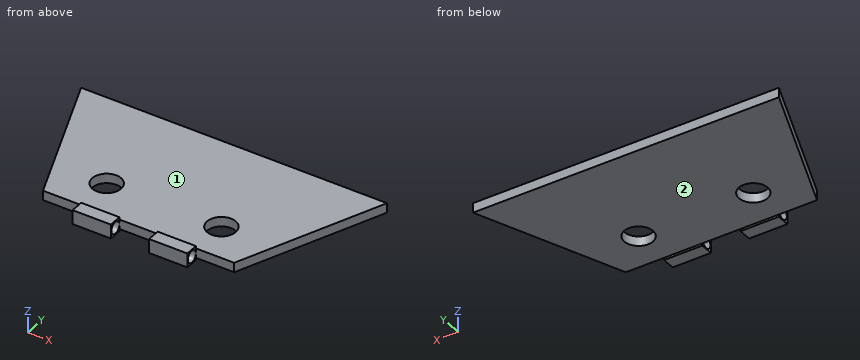
```python
from build123d import *

# Parameters (mm, degrees)
F1_DEPTH = 6.35
F2_W     = 8.614382
F2_H     = 9.368035
F2_R     = 3.988724
F3_DEPTH = 76.2
F4_W     = 25.4
F4_H     = 8.614382
F5_DEPTH = 25.4
F8_D     = 19.05


with BuildPart() as f1:
    # F0 (on Top) → F1 (new body)
    with BuildSketch(Plane.XY):
        Polygon((139.7, 95.249673), (-63.5, 95.249673), (-25.4, 0), (101.6, 0), align=None)
    extrude(amount=F1_DEPTH)

    # F2 (on Right) → F3 (join)
    with BuildSketch(Plane.YZ):
        with Locations((-4.307191, 3.2055)):
            Rectangle(F2_W, F2_H)
        with Locations((-4.046882, 3.205501)):
            Circle(F2_R, mode=Mode.SUBTRACT)
    extrude(amount=F3_DEPTH)

    # F4 (on face) → F5 (cut)
    with BuildSketch(Plane.XY.offset(7.889518)):
        with Locations((38.1, -4.307191)):
            Rectangle(F4_W, F4_H)
    extrude(amount=-F5_DEPTH, mode=Mode.SUBTRACT)

    # F8 (through all)
    with Locations(Plane(origin=(0, 0, 0), x_dir=(1, 0, 0), z_dir=(0, 0, -1))):
        with Locations((0, -25.4), (76.2, -25.4)):
            Hole(F8_D / 2)


solid = f1.part
```
For this review, take the finished solid that the model builds, in its own axes (mm). Face numbers are marked on the shaded views. A direction names the side the tool comes from. Give positions to 0.01 mm unless a question says otherwise; leave off trailing zeros. Write each loop counter-clockwise with the first axis right and the second up, starting at its lowest first coordinate (ties: lowest second). Pieces come first, ordered by that corner, then holes. Notation, with made-up numbers: M -1.5,-30.75 L 17.5,-30.75 A37 ccw 17.5,6.25 Z; hole C -6,57.25 d2. An arc over 180 degrees is marked long. One line per item, written item: value.
1) Take a section at C-C, the plane x = -15. Write out the cut boundary in (y, z).
Results are:
outline: M 0,0 L 95.25,0 L 95.25,6.35 L 0,6.35 Z
2) For the marked faces 1 and 2, list the 3-axis set-ups (+Z, -Z, +X, -X, +Y, -Y) from which the entire face can be reached by the end or side of a thin tool; tool diameter is ignored.
Results are:
face 1: +Z, +X, -X, +Y
face 2: -Z, +X, -X, +Y
3) Take a section at D-D, the plane y = 2. Write out the cut boundary in (x, z).
Results are:
outline: M -26.2,0 L 102.4,0 L 102.4,6.35 L -26.2,6.35 Z
4) Take a section at B-B, the plane x = 70. Write out the cut boundary in (y, z).
Results are:
outline: M -8.61,-1.48 L 0,-1.48 L 0,0 L 18.17,0 L 18.17,6.35 L 0,6.35 L 0,7.89 L -8.61,7.89 Z; M 32.63,0 L 95.25,0 L 95.25,6.35 L 32.63,6.35 Z; hole C -4.05,3.21 d7.98
5) For line 1 (X direction, y = -1, z = 0.5); line 2 (Z direction, x = 30.5, y = 41); line 3 (Y direction, x = 56.5, z = 6), list the stretches that pass through material, from the lowest coordinate up. Write a range as from..to.
Results are:
line 1: x = 0..25.4, 50.8..76.2
line 2: z = 0..6.35
line 3: y = -8.61..-6.89, -1.2..95.25
6) Take a section at A-A, the plane y = 25.4. Write out the cut boundary in (x, z) (3 decimals).
Results are:
outline: M -35.56,0 L -9.525,0 L -9.525,6.35 L -35.56,6.35 Z; M 9.525,0 L 66.675,0 L 66.675,6.35 L 9.525,6.35 Z; M 85.725,0 L 111.76,0 L 111.76,6.35 L 85.725,6.35 Z
7) For P1, Ø1, axis at x = 57.5, y = 48.5, coming from the +Z side; P2, Ø4.5, axis at y = -5, z = 1, coming from the +X side; P3, Ø4, axis at x = 28, z = 1, coming from the -Y side, all flat-tipped, find the tip position at first contact; note any pin that passes through.
Results are:
P1: stops at z = 6.35
P2: stops at x = 76.2
P3: stops at y = 0
